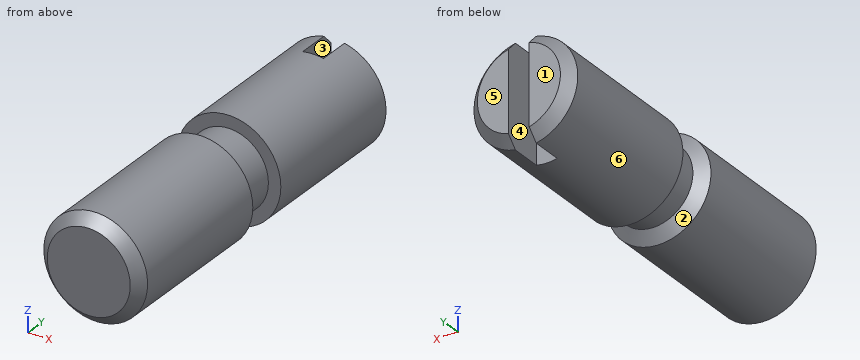
from build123d import *

# Parameters (mm, degrees)
SKIZZE1_R                       = 2.5
AUFSATZ_LINEAR_AUSTRAGEN1_DEPTH = 18
SKIZZE2_W                       = 1
SKIZZE2_H                       = 8.751437557
SCHNITT_LINEAR_AUSTRAGEN1_DEPTH = 2
FASE1_SIZE                      = 0.5


with BuildPart() as part:
    # Skizze1 → Aufsatz-Linear austragen1 (new body)
    with BuildSketch(Plane(origin=(0, 0, 0), x_dir=(1, 0, 0), z_dir=(0, 1, 0))):
        Circle(SKIZZE1_R)
    extrude(amount=AUFSATZ_LINEAR_AUSTRAGEN1_DEPTH)

    # Skizze2 → Schnitt-Linear austragen1 (cut)
    with BuildSketch(Plane(origin=(0, 18, 0), x_dir=(1, 0, 0), z_dir=(0, 1, 0))):
        with Locations((0, -0.571236499)):
            Rectangle(SKIZZE2_W, SKIZZE2_H)
    extrude(amount=-SCHNITT_LINEAR_AUSTRAGEN1_DEPTH, mode=Mode.SUBTRACT)

    # Fase1
    fase1_edges = [part.edges().sort_by_distance(p)[0] for p in [
        (-2.5, 0, 0),
        (1.936491673, 18, 1.58113883),
        (-2.5, 18, 0),
    ]]
    chamfer(fase1_edges, length=FASE1_SIZE)

    # Skizze3 → Schnitt-Rotation1 (revolve, cut)
    with BuildSketch(Plane.XY):
        Polygon((2.5, 10), (1.9, 10), (1.9, 8.404421135), (2.5, 8), align=None)
    revolve(axis=Axis((0, 12.232483269, 0), (0, -1, 0)), mode=Mode.SUBTRACT)


solid = part.part
Model file for the job. Use its own axes, mm. Face numbers are marked on the shaded views. A direction names the side the tool comes from. Round coordinates to 2 decimals unless told otherwise and drop trailing zeros. Order: outer loops, then holes, each group sorted by start corner. A loop starts at its lowest first (then second) coordinate and runs counter-clockwise, first axis right, second up.
(1) Pin check, flat tips, straight feed: pin 1 (3 mm diameter, centred on x = -1, z = 0, fed in from -Y); pin 2 (2 mm diameter, centred on y = 5.5, z = -2, fed in from +X); pin 3 (0.8 mm diameter, centred on x = 0, z = -1, fed in from +Y). Stop position of each tip, or through.
(2) Drill centre lines: line 1 (Y direction, x = -0.35, z = -1.6); line 2 (Y direction, x = -1, z = 1.8); line 3 (Y direction, x = 2.25, z = -0.9). Where is each one in solid material? Low to high.
(3) Band-saw the part on C-C (x = 0). List the corners of the cut face in (y, z), then the cut area to 3 significant figures.
(4) Band-saw the part on D-D (y = 12.5). List the corners of the cut face in (x, z), then the cut area to 3 significant figures.
(5) Pull direction X, two halves, no side cores. Call the marked faces 4, 5 and 6: released by +X, released by -X, zero draft, split by the parting line, or undercut.
(6) Band-saw the part on A-A (z = 0). List the corners of the cut face in (x, y).
(7) 3-axis set-ups, long thin cutter, end or side, ignore diameter. For the marked faces 1, 2 and 3: which of +Z, -Z, +X, -X, +Y, -Y reach the whole face in a straight line?
(8) Band-saw the part on B-B (y = 16.5). List the corners of the cut face in (x, z).
Verdict:
1. pin 1: stops at y = 0
1. pin 2: stops at x = 2.29
1. pin 3: stops at y = 16
2. line 1: y = 0 to 16
2. line 2: y = 0.06 to 8.3, 10 to 17.94
2. line 3: y = 0.42 to 8.05, 10 to 17.58
3. outline: (0, -2) - (0.5, -2.5) - (8, -2.5) - (8.4, -1.9) - (10, -1.9) - (10, -2.5) - (16, -2.5) - (16, 2.5) - (10, 2.5) - (10, 1.9) - (8.4, 1.9) - (8, 2.5) - (0.5, 2.5) - (0, 2) - close
3. area: 77.6 mm2
4. outline: circle Ø5 at (0, 0)
4. area: 19.6 mm2
5. face 4: undercut
5. face 5: zero draft
5. face 6: split by the parting line
6. outline: (-2.5, 0.5) - (-2, 0) - (2, 0) - (2.5, 0.5) - (2.5, 8) - (1.9, 8.4) - (1.9, 10) - (2.5, 10) - (2.5, 17.5) - (2, 18) - (0.5, 18) - (0.5, 16) - (-0.5, 16) - (-0.5, 18) - (-2, 18) - (-2.5, 17.5) - (-2.5, 10) - (-1.9, 10) - (-1.9, 8.4) - (-2.5, 8) - close
7. face 1: +Z, -Z, +X, -X, +Y
7. face 2: none
7. face 3: +Z, -Z, +Y
8. outline: (-0.5, -2.45) - (-0.5, 2.45) arc R2.5 ccw to start; (0.5, -2.45) arc R2.5 ccw to (0.5, 2.45) - close
